```python
from build123d import *

# Parameters (mm, degrees)
Y_KSEKLIK_EKSTR_ZYON1_DEPTH = 10
IZIM2_W                     = 120
IZIM2_H                     = 1
Y_KSEKLIK_EKSTR_ZYON2_DEPTH = 3
IZIM4_W                     = 2
IZIM4_H                     = 10
Y_KSEKLIK_EKSTR_ZYON3_DEPTH = 4
KES_EKSTR_ZYON1_DEPTH       = 33


with BuildPart() as part:
    # Çizim1 → Yükseklik-Ekstrüzyon1 (new body)
    with BuildSketch(Plane.XY):
        Polygon((0, 0), (-120, 0), (-120, -1), (2, -1), (2, 3), (0, 3), align=None)
    y_kseklik_ekstr_zyon1 = extrude(amount=Y_KSEKLIK_EKSTR_ZYON1_DEPTH)

    # Çizim2 → Yükseklik-Ekstrüzyon2 (add)
    with BuildSketch(Plane(origin=(0, 0, 0), x_dir=(1, 0, 0), z_dir=(0, 1, 0))):
        with Locations((-60, -9.5)):
            Rectangle(IZIM2_W, IZIM2_H)
    y_kseklik_ekstr_zyon2 = extrude(amount=Y_KSEKLIK_EKSTR_ZYON2_DEPTH)

    # Çizim4 → Yükseklik-Ekstrüzyon3 (add)
    with BuildSketch(Plane(origin=(0, 3, 0), x_dir=(1, 0, 0), z_dir=(0, 1, 0))):
        with Locations((1, -5)):
            Rectangle(IZIM4_W, IZIM4_H)
    y_kseklik_ekstr_zyon3 = extrude(amount=Y_KSEKLIK_EKSTR_ZYON3_DEPTH)

    # Aynalama1: Yükseklik-Ekstrüzyon1, Yükseklik-Ekstrüzyon2, Yükseklik-Ekstrüzyon3 across plane
    add(y_kseklik_ekstr_zyon1.mirror(Plane(origin=(0, 0, 10), x_dir=(0, 0, 1), z_dir=(1, 0, 0))))
    add(y_kseklik_ekstr_zyon2.mirror(Plane(origin=(0, 0, 10), x_dir=(0, 0, 1), z_dir=(1, 0, 0))))
    add(y_kseklik_ekstr_zyon3.mirror(Plane(origin=(0, 0, 10), x_dir=(0, 0, 1), z_dir=(1, 0, 0))))

    # Çizim5 → Kes-Ekstrüzyon1 (cut)
    with BuildSketch(Plane(origin=(0, 0, 0), x_dir=(-1, 0, 0), z_dir=(0, 0, -1))):
        Polygon((0, 7), (0, -4.162998524), (124.646798912, -4.162998524), (124.646798912, 13.350515485), (0, 13.350515485), align=None)
    extrude(amount=-KES_EKSTR_ZYON1_DEPTH, mode=Mode.SUBTRACT)


solid = part.part
```
Here's how the part is built. I have some questions about the finished solid (model axes, mm). A direction names the side the tool comes from. Give positions to 0.01 mm unless a question says otherwise; leave off trailing zeros. Loops run counter-clockwise (first coordinate to the right, second up) from the corner with the lowest first, then second, coordinate; pieces in that order, holes last. Notation, with made-up numbers: (6, 1.5) -> (29, 1.5) arc R22 ccw to (29, 11.5) -> close; hole circle Ø2 at (22.5, 15.25). An arc over 180 degrees is marked (long way). Use one line per item in the form item = value. Start each with the question number.
1) Please list where these lines run through material, in increasing order: line 1 along X through (y, z) = (4.5, 1); line 2 along Y through (x, z) = (52.5, 9.5); line 3 along Y through (x, z) = (42, 2.5).
2) Imagine slicing it at B-B (y = 5.75). Please give me the cut outline in (x, z), then the cut area to 3 significant figures.
3) Imagine slicing it at C-C (x = 15.5). Please give me the cut outline in (y, z), then the cut area to 3 significant figures.
4) Which directions (+Z, -Z, +X, -X, +Y, -Y) give clear straight access to the entire face, cutting with the end or side of a thin tool? Please do faces 1 (the face through (60, 0, 4)), 2 (the face through (59, -1, 5)).
5) For P1, Ø3, axis at x = 27.5, z = 8, coming from the +Y side; P2, Ø1.5, axis at x = 63.5, y = 1, coming from the -Z side, each with a flat end and sliding along its axis, tell me the tip position at first contact or that it passes through.
6) Imagine slicing it at A-A (z = 3.75). Please give me the cut outline in (x, y), then the cut area to 3 significant figures.
Check values:
q1.line_1 = 0 to 2
q1.line_2 = -1 to 3
q1.line_3 = -1 to 0
q2.outline = (0, 0) -> (2, 0) -> (2, 10) -> (0, 10) -> close
q2.area = 20.0 mm^2
q3.outline = (-1, 0) -> (0, 0) -> (0, 9) -> (3, 9) -> (3, 10) -> (-1, 10) -> close
q3.area = 13.0 mm^2
q4.face_1 = -Z, +X, +Y
q4.face_2 = +Z, -Z, +X, -X, -Y
q5.P1 = 3
q5.P2 = 9
q6.outline = (0, -1) -> (120, -1) -> (120, 0) -> (2, 0) -> (2, 7) -> (0, 7) -> close
q6.area = 134 mm^2
